from build123d import *

# Parameters (mm, degrees)
SKETCH1_W           = 50
SKETCH1_H           = 50
BOSS_EXTRUDE1_DEPTH = 2
SCALE1_SCALE        = 0.5
SCALE2_SCALE        = 0.6
SKETCH3_W           = 2
SKETCH3_H           = 2
BOSS_EXTRUDE2_DEPTH = 2


with BuildPart() as part:
    # Sketch1 → Boss-Extrude1 (new body)
    with BuildSketch(Plane.XY):
        Rectangle(SKETCH1_W, SKETCH1_H)
    extrude(amount=BOSS_EXTRUDE1_DEPTH)

    # Sketch2 → Revolve2 (revolve)
    with BuildSketch(Plane(origin=(0, 0, 0), x_dir=(0, 0, -1), z_dir=(1, 0, 0))):
        with BuildLine():
            Line((0, -20), (0, -18))
            ThreePointArc((0, -18), (12.727922061, -12.727922061), (18, 0))
            Line((18, 0), (20, 0))
            ThreePointArc((20, 0), (14.142135624, -14.142135624), (0, -20))
        make_face()
    revolve(axis=Axis((0, 0, -18), (0, 0, -1)))


with BuildPart() as part_1:
    # Scale1: scaled about (0, 0, -4.005571342)
    add(part.part.scale(SCALE1_SCALE).moved(Location((0, 0, -2.002785671))))


with BuildPart() as part_2:
    # Scale2: scaled about (0, 0, -4.005571342)
    add(part_1.part.scale(SCALE2_SCALE).moved(Location((0, 0, -1.602228537))))

    # Sketch3 → Boss-Extrude2 (add)
    with BuildSketch(Plane(origin=(0, 0, -2.803899939), x_dir=(-1, 0, 0), z_dir=(0, 0, -1))):
        Rectangle(SKETCH3_W, SKETCH3_H)
    extrude(amount=BOSS_EXTRUDE2_DEPTH)


solid = part_2.part
Verification items for the finished model (mm, model axes). A direction names the side the tool comes from. Round coordinates to 2 decimals unless told otherwise and drop trailing zeros. Write each loop counter-clockwise with the first axis right and the second up, starting at its lowest first coordinate (ties: lowest second). Pieces come first, ordered by that corner, then holes.
(1) Section check C-C (x = 3). Enter the section's corners in (y, z).
Returned:
outline: (-7.5, -2.8) - (-5.2, -2.8) arc R5.2 ccw to (5.2, -2.8) - (7.5, -2.8) - (7.5, -2.2) - (-7.5, -2.2) - close; hole (-4.49, -2.8) arc R4.49 ccw to (4.49, -2.8) - close
(2) Section check B-B (y = 1.5). Enter the section's corners in (x, z), plus the area to 3 significant figures.
Returned:
outline: (-7.5, -2.8) - (-5.81, -2.8) arc R5.81 ccw to (5.81, -2.8) - (7.5, -2.8) - (7.5, -2.2) - (-7.5, -2.2) - close; hole (-5.19, -2.8) arc R5.19 ccw to (5.19, -2.8) - close
area: 19.7 mm2
(3) Material ranges on line 1 (Z direction, x = 4.25, y = -5); line 2 (Z direction, x = -4.75, y = 1); line 3 (X direction, y = -1.5, z = -6.5), recorded low to high.
Returned:
line 1: z = -2.8 to -2.2
line 2: z = -6.33 to -5.17, -2.8 to -2.2
line 3: x = -4.48 to -3.64, 3.64 to 4.48
(4) Access from +Z, -Z, +X, -X, +Y, -Y to the whole of each face (thin tool, end or side, straight path). Record for faces 4 (the flat face through (-1, 0, -4)), 5 (the flat face through (-3.44, 5.1, -2.804)).
Returned:
face 4: none
face 5: -Z
(5) Mould release check, pull along X, two halves, no side actions. Record for faces 1 (the flat face through (0, 0, -2.204)), 2 (the flat face through (0, -1, -4)), 3 (the flat face through (0, 1, -4)): pulls with the +X half, pulls with the -X half, needs draft (parallel to the pull), parting line crosses it, or undercut.
Returned:
face 1: needs draft
face 2: undercut
face 3: undercut
(6) Section check D-D (x = -6.25). Enter the section's corners in (y, z), plus the area to 3 significant figures.
Returned:
outline: (-7.5, -2.8) - (7.5, -2.8) - (7.5, -2.2) - (-7.5, -2.2) - close
area: 9.00 mm2
(7) Section check A-A (z = -3.5). Enter the section's corners in (x, y), plus the area to 3 significant figures.
Returned:
outline: circle Ø11.92 at (0, 0); (-1, -1) - (1, -1) - (1, 1) - (-1, 1) - close; hole circle Ø10.71 at (0, 0)
area: 25.5 mm2
(8) Depth check by flat-ended pin: pin 1 Ø3 at (y, z) = (2, -7.5) entering from +X; pin 2 Ø3 at (x, z) = (-2.5, -7) entering from -Y; pin 3 Ø2 at (y, z) = (0, -4) entering from -X. Enter the tip coordinate at first touch or a pass-through.
Returned:
pin 1: stops at x = 4.8
pin 2: stops at y = -4.95
pin 3: stops at x = -6
